Read the model definition and answer for the solid it produces. Units are mm, in the model's axes. A direction names the side the tool comes from. Coordinates: 2 decimals unless noted, no trailing zeros. Write each loop counter-clockwise with the first axis right and the second up, starting at its lowest first coordinate (ties: lowest second). Pieces come first, ordered by that corner, then holes.
(1) The part is cut by section A-A, the plane z = 6.5. State how many separate pieces and enclosed holes the cut face has, and give its area (3 significant figures).
(2) The part is cut by section B-B, the plane x = 37. Determine the outline of the cut face in (y, z), and give its area (3 significant figures).
(3) The part is cut by section D-D, the plane z = 12.5. Determine the outline of the cut face in (x, y).
(4) Given pin 1 (5 mm diameter, centred on x = -4, z = 8, fed in from +Y); pin 2 (5.5 mm diameter, centred on x = 15, z = 7, fed in from -Y); pin 3 (2 mm diameter, centred on x = 21.5, y = -4.5, fed in from +Z); pin 4 (1 mm diameter, centred on y = -1.5, z = 8, fed in from +X), each flat-ended and moving along its own axis, determine where each tip first touches the part or whether it passes through.
(5) Determine the mould class of faces 1 (the flat face through (18, 6, 10.5)), 2 (the flat face through (6.93, -11.24, 6.9)), 3 (the cylindrical face through (8.98, 9.4, 6.9)) for opening direction X: pulls with the +X half, pulls with the -X half, needs draft (parallel to the pull), parting line crosses it, or undercut.
(6) The part is cut by section C-C, the plane x = 2. Determine the outline of the cut face in (y, z).
(7) Straight lines are drawn through the part: line 1 along Y through (x, z) = (16, 8); line 2 along Z through (x, y) = (30, -11); line 3 along Y through (x, z) = (16.5, 9.5). For each, find the intervals that lie inside material, in ascending order.
(8) Which of the six approach directions +Z, -Z, +X, -X, +Y, -Y give full straight-line access (tool end or side, diameter ignored) to faces 4 (the flat face through (15, -12, 10.5)), 5 (the flat face through (40.078, -7.636, 12.226)), 6 (the cylindrical face through (26.2, -8.2, 7)), 7 (the flat face through (18, 4, 7)), 8 (the flat face through (14.29, 15.66, 7.1))?
```python
from build123d import *

# Parameters (mm, degrees)
SKETCH1_R               = 1.65
BOSS_EXTRUDE1_DEPTH     = 14
CUT_EXTRUDE1_DEPTH      = 3.5
CUT_EXTRUDE1_DEPTH_BACK = 3.5
SKETCH4_R               = 4.134785872
CUT_EXTRUDE2_DEPTH      = 15


with BuildPart() as part:
    # Sketch1 → Boss-Extrude1 (new body)
    with BuildSketch(Plane.XY):
        with BuildLine():
            Line((-4.072673183, 12.345579498), (-7.625975393, 11.173383521))
            ThreePointArc((-7.625975393, 11.173383521), (-13.932101619, 14.329478478), (-10.810338029, 20.652670351))
            Line((-10.810338029, 20.652670351), (15.398053767, 29.615676166))
            ThreePointArc((15.398053767, 29.615676166), (20.618433164, 29.610679867), (24.957842791, 26.708627129))
            Line((24.957842791, 26.708627129), (16.98069158, 23.980521824))
            ThreePointArc((16.98069158, 23.980521824), (15.019478176, 19.98069158), (19.01930842, 18.019478176))
            Line((19.01930842, 18.019478176), (26.996459631, 20.747583481))
            ThreePointArc((26.996459631, 20.747583481), (26.541449303, 18.163868162), (25.360666834, 15.821140689))
            ThreePointArc((25.360666834, 15.821140689), (24.782584433, 2.915994941), (36.247809691, -3.035943889))
            ThreePointArc((36.247809691, -3.035943889), (40.533104807, -3.700175716), (44.010342791, -6.291270882))
            Line((44.010342791, -6.291270882), (36.03319158, -9.019376187))
            ThreePointArc((36.03319158, -9.019376187), (34.071978176, -13.019206432), (38.07180842, -14.980419835))
            Line((38.07180842, -14.980419835), (46.048959631, -12.25231453))
            ThreePointArc((46.048959631, -12.25231453), (40.381510061, -20.361577987), (30.691295483, -18.366614362))
            ThreePointArc((30.691295483, -18.366614362), (21.686652044, -14.866973588), (13.021006186, -19.137532201))
            ThreePointArc((13.021006186, -19.137532201), (5.710138119, -19.509709901), (5.863446279, -12.190980179))
            Line((5.863446279, -12.190980179), (8.655248878, -9.699828187))
            ThreePointArc((8.655248878, -9.699828187), (11.258330249, 6.5), (-4.072673183, 12.345579498))
        make_face()
        with Locations((-9.192388155, 15.921683328)):
            Circle(SKETCH1_R, mode=Mode.SUBTRACT)
        with Locations((15.921683328, 9.192388155)):
            Circle(SKETCH1_R, mode=Mode.SUBTRACT)
        with Locations((9.192388155, -15.921683328)):
            Circle(SKETCH1_R, mode=Mode.SUBTRACT)
    extrude(amount=BOSS_EXTRUDE1_DEPTH)

    # Sketch3 → Cut-Extrude1 (cut, two sides)
    with BuildSketch(Plane.XY.offset(7)) as cut_extrude1_sk:
        with BuildLine():
            Line((0, 7), (37.0525, 7))
            Line((37.0525, 7), (37.0525, 4))
            Line((37.0525, 4), (5.744562647, 4))
            ThreePointArc((5.744562647, 4), (6.839579176, -1.490019025), (3.560144623, -6.027053199))
            Line((3.560144623, -6.027053199), (26.472773451, -16.50760099))
            ThreePointArc((26.472773451, -16.50760099), (45.290154871, -3.975495091), (32.268920997, -22.457783645))
            Line((32.268920997, -22.457783645), (-2.911743741, -6.365669516))
            ThreePointArc((-2.911743741, -6.365669516), (-6.839579176, 1.490019025), (0, 7))
        make_face()
    extrude(amount=CUT_EXTRUDE1_DEPTH, mode=Mode.SUBTRACT)
    extrude(cut_extrude1_sk.sketch, amount=-CUT_EXTRUDE1_DEPTH_BACK, mode=Mode.SUBTRACT)

    # Sketch4 → Cut-Extrude2 (cut, through all)
    with BuildSketch(Plane.XY.offset(14)):
        with Locations((18.906044872, -4.601778811)):
            Circle(SKETCH4_R)
        with BuildLine():
            Line((15.638639586, 12.831397119), (12.901157572, 18.566010293))
            ThreePointArc((12.901157572, 18.566010293), (12.545106314, 22.471949344), (14.817713576, 25.668570778))
            Line((14.817713576, 25.668570778), (-5.984422938, 18.554449775))
            ThreePointArc((-5.984422938, 18.554449775), (-5.108522805, 16.659615437), (-5.265913096, 14.578071178))
            ThreePointArc((-5.265913096, 14.578071178), (4.343025459, 14.879117241), (12.281235493, 9.456281234))
            ThreePointArc((12.281235493, 9.456281234), (13.333962642, 11.766529109), (15.638639586, 12.831397119))
        make_face()
    extrude(amount=-CUT_EXTRUDE2_DEPTH, mode=Mode.SUBTRACT)


solid = part.part
```
Computed:
1. separate pieces: 3
1. enclosed holes: 5
1. area: 644 mm2
2. outline: (-21, 0) - (-15.15, 0) - (-15.15, 3.5) - (-21, 3.5) - close; (-21, 10.5) - (-15.15, 10.5) - (-15.15, 14) - (-21, 14) - close; (-8.69, 0) - (-3, 0) - (-3, 3.5) - (-8.69, 3.5) - close; (-8.69, 10.5) - (-3, 10.5) - (-3, 14) - (-8.69, 14) - close
2. area: 80.8 mm2
3. outline: (-10.81, 20.65) arc R5 ccw to (-7.63, 11.17) - (-4.07, 12.35) arc R13 cw to (8.66, -9.7) - (5.86, -12.19) arc R5 ccw (long way) to (13.02, -19.14) arc R12 cw to (30.69, -18.37) arc R9 ccw to (46.05, -12.25) - (38.07, -14.98) arc R3.15 cw to (36.03, -9.02) - (44.01, -6.29) arc R9 ccw to (36.25, -3.04) arc R12 cw to (25.36, 15.82) arc R9 ccw to (27, 20.75) - (19.02, 18.02) arc R3.15 cw to (16.98, 23.98) - (24.96, 26.71) arc R9 ccw to (15.4, 29.62) - close; hole circle Ø3.3 at (-9.19, 15.92); hole (-5.98, 18.55) arc R4.15 cw to (-5.27, 14.58) arc R15.5 cw to (12.28, 9.46) arc R3.65 cw to (15.64, 12.83) - (12.9, 18.57) arc R5.65 cw to (14.82, 25.67) - close; hole circle Ø3.3 at (9.19, -15.92); hole circle Ø3.3 at (15.92, 9.19); hole circle Ø8.27 at (18.91, -4.6)
4. pin 1: stops at y = 23.84
4. pin 2: stops at y = -19.88
4. pin 3: passes through
4. pin 4: stops at x = 30.19
5. face 1: needs draft
5. face 2: pulls with the -X half
5. face 3: undercut
6. outline: (12.85, 0) - (15.37, 0) - (15.37, 14) - (12.85, 14) - close; (21.29, 0) - (25.03, 0) - (25.03, 14) - (21.29, 14) - close
7. line 1: y = -16.59 to -15.02, -11.72 to -7.54, -1.66 to 4, 7 to 7.54, 10.84 to 18.57, 23.43 to 29.77
7. line 2: z = 0 to 3.5, 10.5 to 14
7. line 3: y = -16.3 to -15.24, -11.95 to -7.96, -1.24 to 4, 7 to 7.65, 10.74 to 18.23, 23.77 to 29.87
8. face 4: none
8. face 5: +Z, -Z, +X
8. face 6: +X
8. face 7: +X, -X
8. face 8: +Z, -Z
